Source: CAD feature listing. Evaluate the final solid. Frame: model axes, mm. Face numbers are marked on the shaded views. A direction names the side the tool comes from. Round coordinates to 2 decimals unless told otherwise and drop trailing zeros. Loops run counter-clockwise (first coordinate to the right, second up) from the corner with the lowest first, then second, coordinate; pieces in that order, holes last. Notation, with made-up numbers: (68.25, 29.5) - (124.25, 29.5) arc R30 cw to (124.25, 53.5) - close; hole circle Ø4 at (-13.5, 81.25). An arc over 180 degrees is marked (long way). One line per question, with ' | ' between items. Start each with the question number.
1. Access query for the marked faces 1, 2 and 3. Directions: +Z, -Z, +X, -X, +Y, -Y. A direction counts if a zero-diameter tool reaches every point of the face in a straight line with its end or side. Return the directions, or none.
2. Cut plane D-D (x = 23). Return loops of the section in (y, z), then the cut area to 3 significant figures.
3. Ray query, line 1 (Y direction, x = 44.5, z = 82); line 2 (Y direction, x = 87, z = 61); line 3 (X direction, y = 8, z = 62). Return the intervals inside material, ascending.
4. Pin query (flat end, axial travel): pin 1 (6 mm diameter, centred on x = 34.5, y = 32.5, fed in from +Z); pin 2 (0.8 mm diameter, centred on x = 35, y = 43.5, fed in from -Z); pin 3 (5 mm diameter, centred on x = 37.5, z = 54.5, fed in from +Y). Return the tip coordinate at first contact, or that it passes through.
5. Cut plane A-A (x = 123.5). Return loops of the section in (y, z), then the cut area to 3 significant figures.
6. Cut plane C-C (y = 39). Return loops of the section in (x, z).
7. Cut plane B-B (z = 107). Return loops of the section in (x, y).
```python
from build123d import *

# Parameters (mm, degrees)
BOSS_EXTRUDE1_DEPTH = 44
SHELL1_T            = -2
CUT_EXTRUDE1_START  = -1
CUT_EXTRUDE1_DEPTH  = 1


with BuildPart() as part:
    # Sketch1 → Boss-Extrude1 (new body)
    with BuildSketch(Plane(origin=(0, 0, 0), x_dir=(1, 0, 0), z_dir=(0, 1, 0))):
        with BuildLine():
            Line((0, -150), (0, -50))
            Line((0, -50), (141.421356237, -50))
            ThreePointArc((141.421356237, -50), (86.602540378, -122.474487139), (0, -150))
        make_face()
    extrude(amount=BOSS_EXTRUDE1_DEPTH)

    # Shell1
    shell1_openings = [part.faces().sort_by_distance(p)[0] for p in [
        (56.564232989, 0, 91.421606215),
        (0, 22, 100),
        (70.710678119, 22, 50),
    ]]
    offset(amount=SHELL1_T, openings=shell1_openings, kind=Kind.INTERSECTION)

    # Sketch2 → Cut-Extrude1 (cut)
    with BuildSketch(Plane(origin=(0, 44, 0), x_dir=(1, 0, 0), z_dir=(0, 1, 0)).offset(CUT_EXTRUDE1_START)):
        with BuildLine():
            Line((0, -67.040946117), (131.94510807, -67.040946117))
            ThreePointArc((131.94510807, -67.040946117), (135.889061706, -58.635850029), (139.298241195, -50))
            Line((139.298241195, -50), (0, -50))
            Line((0, -50), (0, -67.040946117))
        make_face()
    extrude(amount=CUT_EXTRUDE1_DEPTH, mode=Mode.SUBTRACT)


solid = part.part
```
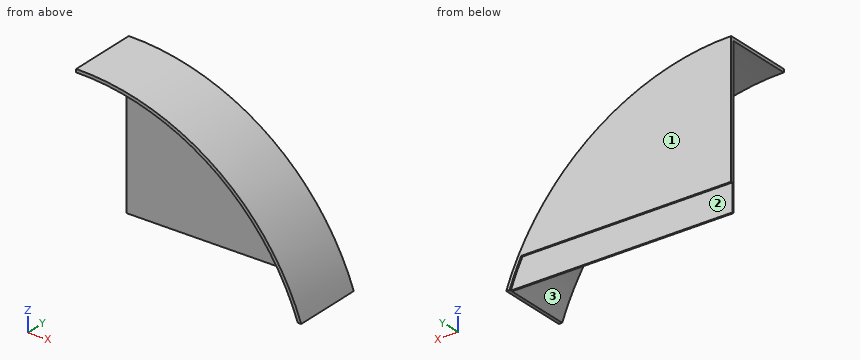
Answers follow:
1) face 1: +Z, -Z, +X, -X, +Y | face 2: -Z, -X, +Y | face 3: -Z, -X, -Y
2) outline: (0, 146.2) - (42, 146.2) - (42, 50) - (43, 50) - (43, 67.04) - (44, 67.04) - (44, 148.23) - (0, 148.23) - close | area: 264 mm2
3) line 1: y = 42 to 44 | line 2: y = 42 to 43 | line 3: x = 134.39 to 136.59
4) pin 1: stops at z = 146.66 | pin 2: stops at z = 67.04 | pin 3: stops at y = 43
5) outline: (0, 81.56) - (42, 81.56) - (42, 50) - (43, 50) - (43, 67.04) - (44, 67.04) - (44, 85.13) - (0, 85.13) - close | area: 203 mm2
6) outline: (0, 148) arc R148 cw to (139.3, 50) - (141.42, 50) arc R150 ccw to (0, 150) - close
7) outline: (0, 42) - (102.25, 42) - (102.25, 0) - (105.12, 0) - (105.12, 44) - (0, 44) - close
